Autodesk Inventor part; units mm, degrees
ref_plane "YZ Plane" through (0, 0, 0) normal (1, 0, 0) x (0, 1, 0)
ref_plane "XZ Plane" through (0, 0, 0) normal (0, 1, 0) x (-1, 0, 0)
ref_plane "XY Plane" through (0, 0, 0) normal (0, 0, 1) x (1, 0, 0)
sketch "Sketch1" plane through (0, 0, 0) normal (0, 0, 1) x (1, 0, 0)
  line L0 (30.125, 0) -> (-30.125, 0)
  line L1 (-16, 18.7) -> (-16, -21.1524) construction
  line L2 (16, 36.5388) -> (16, -18.8821) construction
  line L3 (-16, 18.7) -> (-30.125, 0)
  line L4 (16, 18.7) -> (30.125, 0)
  arc A0 (-4.5, 16.7) -> (-1.5, 16.7) centre (-3, 16.7) ccw
  line L5 (-4.5, 16.7) -> (-4.5, 18.7)
  line L6 (-1.5, 16.7) -> (-1.5, 18.7)
  line L7 (0, 0.7455) -> (0, 23.152) construction
  arc A1 (1.5, 16.7) -> (4.5, 16.7) centre (3, 16.7) ccw
  line L8 (4.5, 16.7) -> (4.5, 18.7)
  line L9 (1.5, 16.7) -> (1.5, 18.7)
  line L10 (4.5, 18.7) -> (16, 18.7)
  line L11 (16, 18.7) -> (4.5, 18.7)
  line L12 (-16, 18.7) -> (-4.5, 18.7)
  line L13 (-1.5, 18.7) -> (1.5, 18.7)
  line L14 (1.5, 18.7) -> (-1.5, 18.7)
  line L15 (-4.5, 18.7) -> (-16, 18.7)
  point P0 (0, 0)
  point P1 (30.125, 18.7)
  point P2 (-30.125, 18.7)
  dimension "d0" = 0
  dimension "d4" = 16
  dimension "d6" = 3
extrude "Extrusion1" add sketch "Sketch1" along normal blind 0.6
chamfer "Chamfer1" distance 0.3 distance2 2 1 edges at (0, 0, 0.6) measured on face at (-10.0417, 0, 0.2)
chamfer "Chamfer2" distance 0.3 distance2 2 1 edges at (0, 0, 0) measured on face at (10.0417, 0, 0.2)
properties part number "Utility Blade (Stanley)"
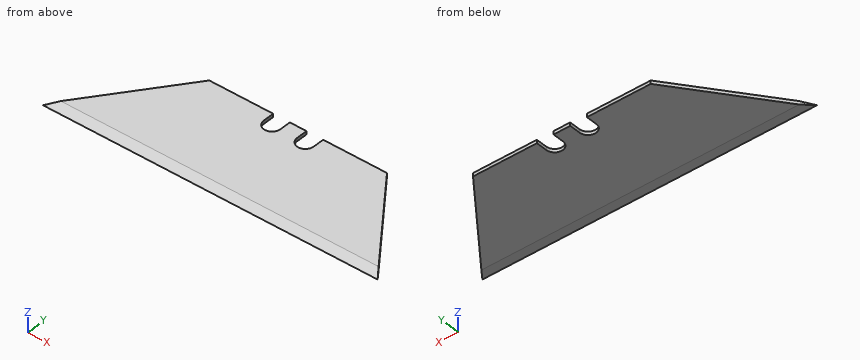
Read the model definition and answer for the solid it produces. Units are mm, in the model's axes. Round coordinates to 2 decimals unless told otherwise and drop trailing zeros. Write each loop counter-clockwise with the first axis right and the second up, starting at its lowest first coordinate (ties: lowest second). Pieces come first, ordered by that corner, then holes. Notation, with made-up numbers: (2.5, 77) - (51.5, 77) arc R27 ccw to (51.5, 104) - close; hole circle Ø11 at (4, -15). An arc over 180 degrees is marked (long way). Use a Markdown table: item, result.
(1) The part is cut by section C-C (z = 0.2). Write down the section's boundary in (x, y), then the cut area to 3 significant figures.
Reported:
| item | result |
|---|---|
| outline | (-29.62, 0.66) - (29.62, 0.66) - (16, 18.7) - (4.5, 18.7) - (4.5, 16.7) arc R1.5 cw to (1.5, 16.7) - (1.5, 18.7) - (-1.5, 18.7) - (-1.5, 16.7) arc R1.5 cw to (-4.5, 16.7) - (-4.5, 18.7) - (-16, 18.7) - close |
| area | 804 mm2 |
(2) Straight lines are drawn through the part: line 1 along X through (y, z) = (10, 0.15); line 2 along X through (y, z) = (4.5, 0.2). For each, find the intervals that lie inside material, in ascending order. Write a range as [from, to].
Reported:
| item | result |
|---|---|
| line 1 | [-22.57, 22.57] |
| line 2 | [-26.73, 26.73] |
(3) The part is cut by section A-A (y = 17.25). Write down the section's boundary in (x, z).
Reported:
| item | result |
|---|---|
| outline | (-17.1, 0) - (-4.5, 0) - (-4.5, 0.6) - (-17.1, 0.6) - close; (-1.5, 0) - (1.5, 0) - (1.5, 0.6) - (-1.5, 0.6) - close; (4.5, 0) - (17.1, 0) - (17.1, 0.6) - (4.5, 0.6) - close |
